Model file for the job. Use its own axes, mm. A direction names the side the tool comes from. Round coordinates to 2 decimals unless told otherwise and drop trailing zeros. Order: outer loops, then holes, each group sorted by start corner. A loop starts at its lowest first (then second) coordinate and runs counter-clockwise, first axis right, second up. Notation, with made-up numbers: (73.5, 76.25) - (111.5, 76.25) arc R25 cw to (111.5, 93.25) - close; hole circle Ø8 at (70, -8). An arc over 180 degrees is marked (long way). Write item = value, one per line. Start each with the question number.
Autodesk Inventor part; units mm, degrees
ref_plane "YZ Plane" through (0, 0, 0) normal (1, 0, 0) x (0, 1, 0)
ref_plane "XZ Plane" through (0, 0, 0) normal (0, 1, 0) x (-1, 0, 0)
ref_plane "XY Plane" through (0, 0, 0) normal (0, 0, 1) x (1, 0, 0)
sketch "Sketch1" plane through (0, 0, 0) normal (0, 0, 1) x (1, 0, 0)
  line L0 (-27.669, 21.4051) -> (50.2215, 21.4051) construction
  line L1 (50.2215, 21.4051) -> (50.2215, -35.1456) construction
  line L2 (50.2215, -35.1456) -> (-27.669, -35.1456) construction
  line L3 (-27.669, -35.1456) -> (-27.669, 21.4051) construction
  line L4 (-25.2081, -35.2295) -> (52.6824, -35.2295) construction
  line L5 (16.9988, 9.3626) -> (27.4291, 9.3626)
  line L6 (30.2909, 8.2443) -> (31.5557, 8.2443)
  line L7 (31.5557, 8.2443) -> (31.5557, 9.1701)
  line L8 (31.5557, 9.1701) -> (33.3477, 10.6493)
  line L9 (33.3477, 10.6493) -> (34.52, 10.6493)
  line L10 (34.52, 10.6493) -> (34.52, 8.2443)
  line L11 (34.52, 8.2443) -> (34.7306, 8.2443)
  line L12 (34.7306, 8.2443) -> (35.1991, 6.7921)
  line L13 (35.1991, 6.7921) -> (22.5878, 6.7921)
  line L14 (22.5878, 6.7921) -> (22.5878, 4.8059)
  line L15 (22.5878, 4.8059) -> (19.0643, 4.0103)
  line L16 (19.0643, 4.0103) -> (17.8875, 2.5188)
  line L17 (17.8875, 2.5188) -> (15.4819, 2.5188)
  line L18 (16.9988, 9.3626) -> (16.9988, 5.4381)
  arc A0 (15.4819, 2.5188) -> (16.9988, 5.4381) centre (13.4312, 5.4381) ccw
  arc A1 (27.4291, 9.3626) -> (30.2909, 8.2443) centre (30.2909, 12.4655) ccw
  line L19 (36.8494, 6.7921) -> (35.3044, 6.7921)
  line L20 (36.8494, 6.7921) -> (35.3044, 6.7921) construction
  line L21 (36.8494, 6.7921) -> (35.3044, 6.7921) construction
  point P0 (0, 0)
  point P1 (26.4448, 6.7921)
  dimension "d1" = 77.8905
  dimension "d2" = 77.8905
extrude "Plate1" add sketch "Sketch1" along normal blind 1.5
equation "\"d2\" = d1"
equation "\"d31\" = Thickness"
equation "\"BendRadius\" = Thickness"
equation "\"BendReliefWidth\" = Thickness"
equation "\"BendReliefDepth\" = 0.5 * Thickness"
equation "\"CornerReliefSize\" = 4 * Thickness"
equation "\"MinimumRemnant\" = 2 * Thickness"
equation "\"TransitionRadius\" = BendRadius"
equation "\"JacobiRadiusSize\" = BendRadius"
equation "\"GapSize\" = Thickness"
properties part number "inner slider"
Item 1: Drop a flat-ended pin along its axis: pin 1 (0.8 mm diameter, centred on y = 8, z = 1, fed in from -X). Give the stop position or say it passes through.
Item 2: Saw through at B-B, the plane y = 7.25. Give the cut face in (x, z), then the cut area to 3 significant figures.
Item 3: Saw through at A-A, the plane z = 1.2. Give the cut face in (x, y).
Item 4: Probe L1, parallel to Y at x = 34, z = 0.75; L2, parallel to Y at x = 17.5, z = 0.95; L3, parallel to X at y = 5.25, z = 0.65. List the from-to ranges inside material, lowest first.
Item 5: Which spindle directions (+Z, -Z, +X, -X, +Y, -Y) get a long thin tool onto all of the face, cutting with end or side? Do faces 4 (the face through (31, 8.244, 1)), 5 (the face through (34.52, 9, 1)), 6 (the face through (25, 8, 1.5)), 7 (the face through (29, 6.792, 1)). Say none if no direction does.
Item 6: Saw through at C-C, the plane x = 29.5. Give the cut face in (y, z), then the cut area to 3 significant figures.
Item 7: Mould opens along X. For faces 1 (the face through (28.775, 8.526, 0.74)), 2 (the face through (16.999, 7, 1)), 3 (the face through (22, 9.363, 1)) say: +X half, -X half, draft (parallel to the pull), parting line (faces both ways), or undercut.
Check sheet entries:
q1.pin_1 = 17
q2.outline = (17, 0) - (35.05, 0) - (35.05, 1.5) - (17, 1.5) - close
q2.area = 27.1 mm2
q3.outline = (15.48, 2.52) - (17.89, 2.52) - (19.06, 4.01) - (22.59, 4.81) - (22.59, 6.79) - (35.2, 6.79) - (34.73, 8.24) - (34.52, 8.24) - (34.52, 10.65) - (33.35, 10.65) - (31.56, 9.17) - (31.56, 8.24) - (30.29, 8.24) arc R4.22 cw to (27.43, 9.36) - (17, 9.36) - (17, 5.44) arc R3.57 cw to start
q4.L1 = 6.79 to 10.65
q4.L2 = 2.52 to 9.36
q4.L3 = 16.99 to 22.59
q5.face_4 = +Z, -Z, +Y
q5.face_5 = +Z, -Z, +X, +Y
q5.face_6 = +Z, +X, -X, +Y, -Y
q5.face_7 = +Z, -Z, +X, -Y
q6.outline = (6.79, 0) - (8.32, 0) - (8.32, 1.5) - (6.79, 1.5) - close
q6.area = 2.29 mm2
q7.face_1 = undercut
q7.face_2 = -X half
q7.face_3 = draft
